The model under review builds one solid part; all positions refer to its coordinate system, in mm. A direction names the side the tool comes from. Give positions to 0.01 mm unless a question says otherwise; leave off trailing zeros. Order: outer loops, then holes, each group sorted by start corner. A loop starts at its lowest first (then second) coordinate and runs counter-clockwise, first axis right, second up. Notation, with made-up numbers: (28, -30.75) - (32, -30.75) arc R29 ccw to (32, 8.25) - close; hole circle Ø4 at (5, 16.5). An arc over 180 degrees is marked (long way). Use CSV: the item, a comma, the result in double quotes.
```python
from build123d import *

# Parameters (mm, degrees)
F0_R           = 5
F1_DEPTH       = 90
F3_R           = 5
F8_R           = 2
F9_DEPTH       = 25
F9_DEPTH_BACK  = 3
F11_R          = 5
F11_R_2        = 4
F12_DEPTH      = 4
F14_R          = 1
F15_DEPTH      = 5.001
F15_DEPTH_BACK = 5.001


with BuildPart() as f1:
    # F0 (on Front) → F1 (new body)
    with BuildSketch(Plane.XZ):
        Circle(F0_R)
    extrude(amount=F1_DEPTH)

    # F4: sweep along a path in F2
    with BuildLine(Plane.XY) as f4_path:
        ThreePointArc((0, 0), (45, -45), (0, -90))
    # F3 (on Right) → F4 (sweep)
    with BuildSketch(Plane.YZ):
        with Locations((-90, 0)):
            Circle(F3_R)
    sweep(path=f4_path.line)

    # F1_face (on face) → F5 (revolve)
    with BuildSketch(Plane(origin=(-2.122066, 0, 0), x_dir=(1, 0, 0), z_dir=(0, 1, 0))):
        with BuildLine():
            Line((2.122066, -5), (2.122066, 5))
            ThreePointArc((2.122066, 5), (-2.877934, 0), (2.122066, -5))
        make_face()
    revolve(axis=Axis((0, 0, 0), (0, 0, 1)))

    # F7: F1 across plane


with BuildPart() as f1_1:
    add(f1.part)
    add(f1.part.mirror(Plane.XZ.offset(45)))

    # F8 (on Top) → F9 (cut, two sides)
    with BuildSketch(Plane.XY) as f9_sk:
        Circle(F8_R)
        with Locations((0, -90)):
            Circle(F8_R)
        with Locations((31.819805, -76.819805)):
            Circle(F8_R)
        with Locations((45, -45)):
            Circle(F8_R)
        with Locations((31.819805, -13.180195)):
            Circle(F8_R)
        with Locations((0, -45)):
            Circle(F8_R)
    extrude(amount=F9_DEPTH, mode=Mode.SUBTRACT)
    extrude(f9_sk.sketch, amount=-F9_DEPTH_BACK, mode=Mode.SUBTRACT)

    # F11 (on offset) → F12 (cut, symmetric)
    with BuildSketch(Plane.XZ.offset(67.5)):
        Circle(F11_R)
        Circle(F11_R_2, mode=Mode.SUBTRACT)
    extrude(amount=F12_DEPTH, both=True, mode=Mode.SUBTRACT)

    # F13: F1 across plane


with BuildPart() as f1_2:
    add(f1_1.part)
    add(f1_1.part.mirror(Plane.XZ.offset(45)), mode=Mode.INTERSECT)

    # F14 (on Top) → F15 (cut, two sides)
    with BuildSketch(Plane.XY) as f15_sk:
        with Locations((17.220754, -86.574579)):
            Circle(F14_R)
        with Locations((41.574579, -62.220754)):
            Circle(F14_R)
        with Locations((41.574579, -27.779246)):
            Circle(F14_R)
        with Locations((17.220754, -3.425421)):
            Circle(F14_R)
    extrude(amount=F15_DEPTH, mode=Mode.SUBTRACT)
    extrude(f15_sk.sketch, amount=-F15_DEPTH_BACK, mode=Mode.SUBTRACT)


solid = f1_2.part
```
Item 1: Clearance check with flat-ended pins moving along their axes: pin 1 (1.8 mm diameter, centred on x = 41.57, y = -62.22, fed in from +Z); pin 2 (1.2 mm diameter, centred on x = -1, y = -89.5, fed in from +Z); pin 3 (1 mm diameter, centred on x = 39, z = -2, fed in from -Y); pin 4 (10 mm diameter, centred on x = 30.5, y = -67.5, fed in from -Z). State where each tip first meets the part, or that it passes through.
Results list:
pin 1,"passes through"
pin 2,"stops at z = -3"
pin 3,"stops at y = -76.32"
pin 4,"stops at z = -4.54"
Item 2: Tool access review of faces 1 (the face through (-0.867, -22.556, -3.905)), 2 (the face through (0, -2, 1)): name each direction out of +Z, -Z, +X, -X, +Y, -Y from which nothing blocks a thin tool from reaching the whole face with its end or side.
Results list:
face 1,"none"
face 2,"+Z"
Item 3: Wall thickness on L1, parallel to X at y = -27.5, z = 1.75; L2, parallel to Y at x = 10, z = -4.25; L3, parallel to X at y = -58, z = 1.25: over which ranges is each line inside the solid? List them lowest first.
Results list:
L1,"x = -4.68 to 4.68, 36.32 to 40.61, 42.53 to 46.5"
L2,"y = -91.57 to -86.17, -3.83 to 1.57"
L3,"x = -4.84 to 4.84, 38 to 48.12"
Item 4: Take a section at A-A, the plane y = -45. Give the boundary of the cut face in (x, z), and give its area (3 significant figures).
Results list:
outline,"(-2, -3) - (-2, 4.58) arc R5 ccw (long way) to (2, 4.58) - (2, -3) - close; (43, -3) - (43, 4.58) arc R5 ccw (long way) to (47, 4.58) - (47, -3) - close"
area,"94.2 mm2"
Item 5: Take a section at B-B, the plane z = 2.5. State how many separate pieces and enclosed holes the cut face has, and give its area (3 significant figures).
Results list:
separate pieces,"1"
enclosed holes,"11"
area,"1,870 mm2"
